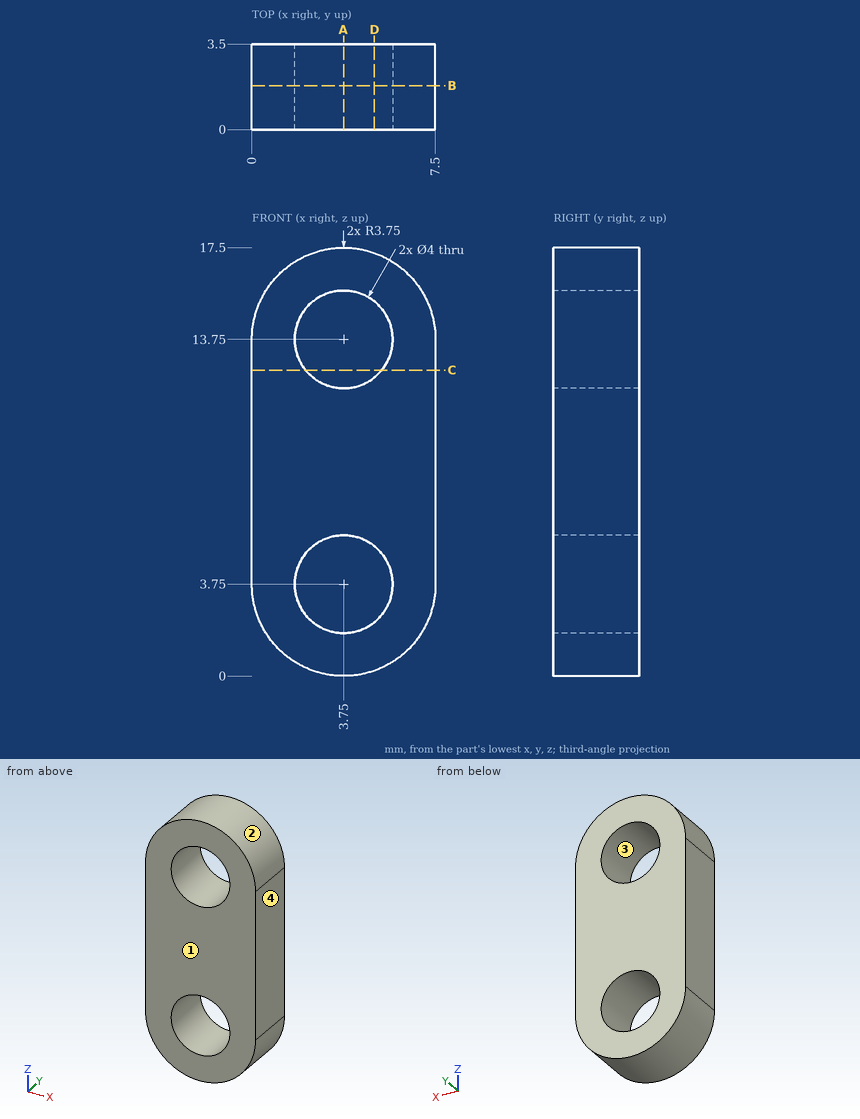
Design review of the part shown in the three views and the two pictorial views. Dimensions are in mm from the part's minimum x, y and z. Give positions to 0.01 mm unless a question says otherwise; leave off trailing zeros. Write each loop counter-clockwise with the first axis right and the second up, starting at its lowest first coordinate (ties: lowest second). Pieces come first, ordered by that corner, then holes.
(1) Mouldability with a two-part tool opening along X and no side actions: class the marked faces 1, 2, 3 and 4 as +X half, -X half, draft (parallel to the pull), parting line (faces both ways), or undercut.
Checked values:
face 1: draft
face 2: parting line
face 3: undercut
face 4: +X half
(2) Add section A-A (x = 3.75). Give the boundary of the cut face in (y, z).
Checked values:
outline: (0, 0) - (3.5, 0) - (3.5, 1.75) - (0, 1.75) - close; (0, 5.75) - (3.5, 5.75) - (3.5, 11.75) - (0, 11.75) - close; (0, 15.75) - (3.5, 15.75) - (3.5, 17.5) - (0, 17.5) - close
(3) Clearance check with flat-ended pins moving along their axes: pin 1 Ø2.5 at (x, z) = (3.75, 3.75) entering from -Y; pin 2 Ø1.5 at (x, y) = (2, 1.5) entering from +Z; pin 3 Ø2 at (x, y) = (5, 3) entering from +Z. State where each tip first meets the part, or that it passes through.
Checked values:
pin 1: passes through
pin 2: stops at z = 17.36
pin 3: stops at z = 17.49
(4) Wall thickness on line 1 along Z through (x, y) = (3.75, 1.5); line 2 along X through (y, z) = (2, 13.75); line 3 along Z through (x, y) = (4.5, 1.85): over which ranges is each line inside the solid? List them lowest first.
Checked values:
line 1: z = 0 to 1.75, 5.75 to 11.75, 15.75 to 17.5
line 2: x = 0 to 1.75, 5.75 to 7.5
line 3: z = 0.08 to 1.9, 5.6 to 11.9, 15.6 to 17.42
(5) Add section C-C (z = 12.5). Give the boundary of the cut face in (x, y).
Checked values:
outline: (0, 0) - (2.19, 0) - (2.19, 3.5) - (0, 3.5) - close; (5.31, 0) - (7.5, 0) - (7.5, 3.5) - (5.31, 3.5) - close
(6) Add section D-D (x = 5). Give the boundary of the cut face in (y, z).
Checked values:
outline: (0, 0.21) - (3.5, 0.21) - (3.5, 2.19) - (0, 2.19) - close; (0, 5.31) - (3.5, 5.31) - (3.5, 12.19) - (0, 12.19) - close; (0, 15.31) - (3.5, 15.31) - (3.5, 17.29) - (0, 17.29) - close
(7) Add section B-B (y = 1.8). Give the boundary of the cut face in (x, z), and give its area (3 significant figures).
Checked values:
outline: (0, 3.75) arc R3.75 ccw to (7.5, 3.75) - (7.5, 13.75) arc R3.75 ccw to (0, 13.75) - close; hole circle Ø4 at (3.75, 3.75); hole circle Ø4 at (3.75, 13.75)
area: 94.0 mm2
